Source: CAD feature listing. Evaluate the final solid. Frame: model axes, mm. A direction names the side the tool comes from. Coordinates: 2 decimals unless noted, no trailing zeros. Loops run counter-clockwise (first coordinate to the right, second up) from the corner with the lowest first, then second, coordinate; pieces in that order, holes last.
from build123d import *

# Parameters (mm, degrees)
SKETCH1_W                                            = 152.4
SKETCH1_H                                            = 101.6
BOSS_EXTRUDE1_DEPTH                                  = 12.7
CBORE_FOR_1_4_BINDING_HEAD_MACHINE_SCREW_D           = 6.858
CBORE_FOR_1_4_BINDING_HEAD_MACHINE_SCREW_CBORE_D     = 14.2875
CBORE_FOR_1_4_BINDING_HEAD_MACHINE_SCREW_CBORE_DEPTH = 6.35
F_1_4_0_25_DIAMETER_HOLE1_D                          = 6.858
CUT_EXTRUDE1_DEPTH                                   = 6.35


with BuildPart() as part:
    # Sketch1 → Boss-Extrude1 (new body)
    with BuildSketch(Plane(origin=(0, 0, 0), x_dir=(1, 0, 0), z_dir=(0, 1, 0))):
        Rectangle(SKETCH1_W, SKETCH1_H)
    extrude(amount=BOSS_EXTRUDE1_DEPTH)

    # CBORE for 1/4 Binding Head Machine Screw1 (through all)
    with Locations(Plane(origin=(0, 12.7, 0), x_dir=(1, 0, 0), z_dir=(0, 1, 0))):
        with Locations((-38.1, 38.1), (38.1, 38.1), (38.1, -38.1), (-38.1, -38.1)):
            CounterBoreHole(CBORE_FOR_1_4_BINDING_HEAD_MACHINE_SCREW_D / 2, CBORE_FOR_1_4_BINDING_HEAD_MACHINE_SCREW_CBORE_D / 2, CBORE_FOR_1_4_BINDING_HEAD_MACHINE_SCREW_CBORE_DEPTH)

    # 1/4 (0.25) Diameter Hole1 (through all)
    with Locations(Plane(origin=(0, 12.7, 0), x_dir=(1, 0, 0), z_dir=(0, 1, 0))):
        with Locations((0, 0), (25.4, 0), (50.8, 0), (-25.4, 0), (-50.8, 0)):
            Hole(F_1_4_0_25_DIAMETER_HOLE1_D / 2)

    # Sketch6 → Cut-Extrude1 (cut)
    with BuildSketch(Plane.XZ):
        Polygon((19.90725, -3.171240691), (25.4, -6.342481382), (30.89275, -3.171240691), (30.89275, 3.171240691), (25.4, 6.342481382), (19.90725, 3.171240691), align=None)
        Polygon((50.8, 6.342481382), (45.30725, 3.171240691), (45.30725, -3.171240691), (50.8, -6.342481382), (56.29275, -3.171240691), (56.29275, 3.171240691), align=None)
        Polygon((-5.49275, -3.171240691), (0, -6.342481382), (5.49275, -3.171240691), (5.49275, 3.171240691), (0, 6.342481382), (-5.49275, 3.171240691), align=None)
        Polygon((-30.89275, -3.171240691), (-25.4, -6.342481382), (-19.90725, -3.171240691), (-19.90725, 3.171240691), (-25.4, 6.342481382), (-30.89275, 3.171240691), align=None)
        Polygon((-56.29275, -3.171240691), (-50.8, -6.342481382), (-45.30725, -3.171240691), (-45.30725, 3.171240691), (-50.8, 6.342481382), (-56.29275, 3.171240691), align=None)
    extrude(amount=-CUT_EXTRUDE1_DEPTH, mode=Mode.SUBTRACT)


solid = part.part
Q1. Line query: line 1 along X through (y, z) = (8.25, -33); line 2 along Z through (x, y) = (-38.1, 9.5); line 3 along Z through (x, y) = (38.1, 4.25). Output: solid intervals per line, ascending.
Q2. Section A-A, the plane z = -38.1. Return the cut outline in (x, y).
Q3. Access query for faces 1 (the cylindrical face through (36.551, 9.569, 45.074)), 2 (the cylindrical face through (-35.573, 3.131, 35.783)), 3 (the flat face through (2.785, 3.131, 4.735)). Directions: +Z, -Z, +X, -X, +Y, -Y. A direction counts if a zero-diameter tool reaches every point of the face in a straight line with its end or side. Return the directions, or none.
Q4. Draft query along X for faces 4 (the flat face through (-1, 6, -50.8)), 5 (the flat face through (36, 6.35, -35)), 6 (the cylindrical face through (0.74, 9.48, 3.35)). Return one class per face: +X half, -X half, draft (parallel to the pull), parting line (faces both ways), or undercut.
Q5. Section C-C, the plane y = 4.25. Count the separate pieces of the cut face and the enclosed holes in it, plus the area to 3 significant figures.
Q6. Contact query for flat-ended pins moving along their axis: pin 1 Ø3.5 at (x, z) = (-49, -1.5) entering from -Y; pin 2 Ø11.5 at (x, z) = (-38.1, 38.1) entering from +Y. Output: stop coordinate, or through.
Q7. Section B-B, the plane x = -38.1. Return the cut outline in (y, z).
Derived:
1. line 1: x = -76.2 to -43.1, -33.1 to 33.1, 43.1 to 76.2
1. line 2: z = -50.8 to -45.24, -30.96 to 30.96, 45.24 to 50.8
1. line 3: z = -50.8 to -41.53, -34.67 to 34.67, 41.53 to 50.8
2. outline: (-76.2, 0) - (-41.53, 0) - (-41.53, 6.35) - (-45.24, 6.35) - (-45.24, 12.7) - (-76.2, 12.7) - close; (-34.67, 0) - (34.67, 0) - (34.67, 6.35) - (30.96, 6.35) - (30.96, 12.7) - (-30.96, 12.7) - (-30.96, 6.35) - (-34.67, 6.35) - close; (41.53, 0) - (76.2, 0) - (76.2, 12.7) - (45.24, 12.7) - (45.24, 6.35) - (41.53, 6.35) - close
3. face 1: +Y
3. face 2: +Y, -Y
3. face 3: -Y
4. face 4: draft
4. face 5: undercut
4. face 6: undercut
5. separate pieces: 1
5. enclosed holes: 9
5. area: 14,800 mm2
6. pin 1: stops at y = 6.35
6. pin 2: stops at y = 6.35
7. outline: (0, -50.8) - (12.7, -50.8) - (12.7, -45.24) - (6.35, -45.24) - (6.35, -41.53) - (0, -41.53) - close; (0, -34.67) - (6.35, -34.67) - (6.35, -30.96) - (12.7, -30.96) - (12.7, 30.96) - (6.35, 30.96) - (6.35, 34.67) - (0, 34.67) - close; (0, 41.53) - (6.35, 41.53) - (6.35, 45.24) - (12.7, 45.24) - (12.7, 50.8) - (0, 50.8) - close
